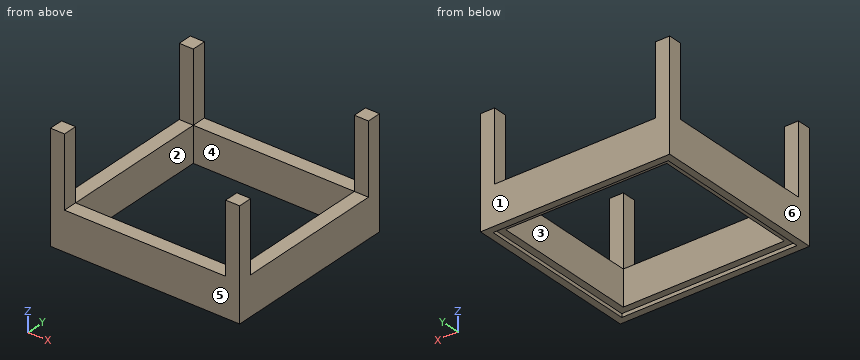
from build123d import *

# Parameters (mm, degrees)
F1_DEPTH = 1.27
F2_W     = 68.58
F2_H     = 64.22644
F2_W_2   = 63.5
F2_H_2   = 59.14644
F2_W_3   = 58.42
F2_H_3   = 54.06644
F3_DEPTH = 12.7
F4_W     = 5.08
F4_H     = 5.08
F5_DEPTH = 25.4


with BuildPart() as f1:
    # F0 (on Top) → F1 (new body)
    with BuildSketch(Plane.XY):
        Polygon((0, -2.54), (0, 0), (0, 59.14644), (63.5, 59.14644), (63.5, 61.68644), (-2.54, 61.68644), (-2.54, 0), (-2.54, -2.54), align=None)
        Polygon((63.5, 0), (0, 0), (0, -2.54), (66.04, -2.54), (66.04, 59.14644), (66.04, 61.68644), (63.5, 61.68644), (63.5, 59.14644), align=None)
    extrude(amount=F1_DEPTH)

    # F2 (on face) → F3 (join)
    with BuildSketch(Plane.XY.offset(1.27)):
        with Locations((31.75, 29.57322)):
            Rectangle(F2_W, F2_H)
        with Locations((31.75, 29.57322)):
            Rectangle(F2_W_2, F2_H_2, mode=Mode.SUBTRACT)
        with Locations((31.75, 29.57322)):
            Rectangle(F2_W_2, F2_H_2)
        with Locations((31.75, 29.57322)):
            Rectangle(F2_W_3, F2_H_3, mode=Mode.SUBTRACT)
    extrude(amount=F3_DEPTH)

    # F4 (on face) → F5 (join)
    with BuildSketch(Plane.XY.offset(13.97)):
        with Locations((0, 59.14644)):
            Rectangle(F4_W, F4_H)
        Rectangle(F4_W, F4_H)
        with Locations((63.5, 0)):
            Rectangle(F4_W, F4_H)
        with Locations((63.5, 59.14644)):
            Rectangle(F4_W, F4_H)
    extrude(amount=F5_DEPTH)


solid = f1.part
Input: part model. Units: mm. Frame: model coordinates. Face numbers are marked on the shaded views. A direction names the side the tool comes from. Round coordinates to 2 decimals unless told otherwise and drop trailing zeros. Order: outer loops, then holes, each group sorted by start corner. A loop starts at its lowest first (then second) coordinate and runs counter-clockwise, first axis right, second up. Notation, with made-up numbers: (88, -37.5) - (94, -37.5) arc R26 cw to (94, -19.5) - close; hole circle Ø9 at (3, 34). An arc over 180 degrees is marked (long way). Answer as a JSON object with one key per item and string values. Group by question number.
(1) Cut plane C-C (y = 3.5). Return loops of the section in (x, z), then the cut area to 3 significant figures.
(2) Reachability of the marked faces 1 and 2 from +Z, -Z, +X, -X, +Y, -Y: full face, straight path, thin tool, end or side. Return the list, or none.
(3) Draft query along X for the marked faces 3, 4, 5 and 6. Return one class per face: released by +X, released by -X, zero draft, split by the parting line, or undercut.
(4) Material intervals for probe 1 along X at (y, z) = (33.5, 10); probe 2 along Y at (x, z) = (63.5, 30.5); probe 3 along Z at (x, y) = (61, 29.5), sorted ascending. Write a range as from..to.
(5) Cut plane A-A (z = 36). Return loops of the section in (x, y), then the cut area to 3 significant figures.
(6) Pin query (flat end, axial travel): P1, Ø5.5, axis at x = 17.5, y = 60.5, coming from the +Z side; P2, Ø12, axis at x = 39.5, y = 48, coming from the -Z side. Return the tip coordinate at first contact, or that it passes through.
(7) Cut plane B-B (x = 25.5). Return loops of the section in (y, z), then the cut area to 3 significant figures.
Here are the results:
{
 "1": {"outline": "(-2.54, 0) - (0, 0) - (0, 1.27) - (2.54, 1.27) - (2.54, 13.97) - (-2.54, 13.97) - close; (60.96, 1.27) - (63.5, 1.27) - (63.5, 0) - (66.04, 0) - (66.04, 13.97) - (60.96, 13.97) - close", "area": "135 mm^2"},
 "2": {"face 1": "+Z, -Z, +X, -X, +Y", "face 2": "+Z, -Z"},
 "3": {"face 3": "undercut", "face 4": "undercut", "face 5": "zero draft", "face 6": "released by -X"},
 "4": {"probe 1": "x = -2.54..2.54, 60.96..66.04", "probe 2": "y = -2.54..2.54, 56.61..61.69", "probe 3": "z = 1.27..13.97"},
 "5": {"outline": "(-2.54, -2.54) - (2.54, -2.54) - (2.54, 2.54) - (-2.54, 2.54) - close; (-2.54, 56.61) - (2.54, 56.61) - (2.54, 61.69) - (-2.54, 61.69) - close; (60.96, -2.54) - (66.04, -2.54) - (66.04, 2.54) - (60.96, 2.54) - close; (60.96, 56.61) - (66.04, 56.61) - (66.04, 61.69) - (60.96, 61.69) - close", "area": "103 mm^2"},
 "6": {"P1": "stops at z = 13.97", "P2": "passes through"},
 "7": {"outline": "(-2.54, 0) - (0, 0) - (0, 1.27) - (2.54, 1.27) - (2.54, 13.97) - (-2.54, 13.97) - close; (56.61, 1.27) - (59.15, 1.27) - (59.15, 0) - (61.69, 0) - (61.69, 13.97) - (56.61, 13.97) - close", "area": "135 mm^2"}
}
